Autodesk Inventor part; units mm, degrees
ref_plane "YZ Plane" through (0, 0, 0) normal (1, 0, 0) x (0, 1, 0)
ref_plane "XZ Plane" through (0, 0, 0) normal (0, 1, 0) x (-1, 0, 0)
ref_plane "XY Plane" through (0, 0, 0) normal (0, 0, 1) x (1, 0, 0)
sketch "Szkic1" plane through (0, 0, 0) normal (0, 0, 1) x (1, 0, 0)
  line L0 (9.9, 0) -> (9.9, 2)
  line L1 (9.9, 2) -> (1.4, 2)
  line L2 (1.4, 2) -> (0.4, 3)
  line L3 (0.4, 3) -> (0, 3)
  arc A0 (0, 3) -> (-1.4487, 0) centre (8.1549, -2.7877) ccw
  line L4 (-1.1, 1) -> (9.9, 1) construction
  line L5 (-1.4487, 0) -> (0, 0)
  line L6 (9.9, 0) -> (0, 0)
  dimension "d1" = 11
  dimension "d2" = 1.1
  dimension "d3" = 10
  dimension "d9" = 2.5
  dimension "d10" = 45
  dimension "d11" = 1
  dimension "d12" = 3
revolve "Obrót1" add sketch "Szkic1" angle 360 about axis through (9.9, 0, 0) along (-1, 0, 0)
sketch "Szkic2" plane through (9.9, 0, 0) normal (1, 0, 0) x (0, 0, -1)
  circle A0 centre (0, 0) radius 2
  line L0 (-1.1303, -1.65) -> (1.1303, -1.65)
  line L1 (1.65, -1.1303) -> (1.65, 1.1303)
  line L2 (1.1303, 1.65) -> (-1.1303, 1.65)
  line L3 (-1.65, 1.1303) -> (-1.65, -1.1303)
  line L4 (-1.65, -1.65) -> (1.65, 1.65) construction
  line L5 (1.65, -1.65) -> (-1.65, 1.65) construction
  dimension "d14" = 3.3
  dimension "d15" = 3.3
extrude "Wyciągnięcie proste2" cut sketch "Szkic2" against normal blind 4 contours A0 L1 | L2 A0 | A0 L0 | L3 A0
sketch "Szkic3" plane through (9.9, -1.1303, -1.65) normal (1, 0, 0) x (0, 0, -1)
  line L0 (-2.7803, -0.5197) -> (-0.5197, -0.5197)
  arc A0 (-0.5197, -0.5197) -> (0, 0) centre (-1.65, 1.1303) ccw
  line L1 (0, 0) -> (0, 2.2605)
  arc A1 (0, 2.2605) -> (-0.5197, 2.7803) centre (-1.65, 1.1303) ccw
  line L2 (-0.5197, 2.7803) -> (-2.7803, 2.7803)
  arc A2 (-2.7803, 2.7803) -> (-3.3, 2.2605) centre (-1.65, 1.1303) ccw
  line L3 (-3.3, 2.2605) -> (-3.3, 0)
  arc A3 (-3.3, 0) -> (-2.7803, -0.5197) centre (-1.65, 1.1303) ccw
hole "Otwór1" at (9.9, 0, 0) direction (-1, 0, 0) diameter 1.8 end through all counterbore diameter 2.4 counterbore depth 2.5
chamfer "Faza1" distance 0.25 angle 45 1 edges at (7.4, 0, 0.9)
chamfer "Faza2" distance 0.25 angle 45 2 edges at (-1.1403, -0.6363, 0.6365) (-1.1403, 0.6364, -0.6364)
sketch "Szkic5" plane through (0, 0, 0) normal (0, 1, 0) x (-1, 0, 0)
  line L0 (0, 3) -> (0, -3) construction
  line L1 (1.0546, -0.55) -> (-0.0454, -0.55)
  line L2 (-0.0454, -0.55) -> (-0.0454, 0.55)
  line L3 (-0.0454, 0.55) -> (1.0546, 0.55)
  line L4 (1.0546, 0.55) -> (1.0546, -0.55)
  line L5 (1.0546, -0.55) -> (-0.0454, 0.55) construction
  line L6 (-0.0454, -0.55) -> (1.0546, 0.55) construction
  point P0 (0, 0)
  point P1 (0.5046, 0)
  dimension "d33" = 1.1
  dimension "d34" = 1.1
extrude "Wyciągnięcie proste3" cut sketch "Szkic5" along normal through all both and the other way through all
thread "Gwint1"
properties part number "Nypel_szprychy" material "Aluminium AW-7020"
Here's how the part is built. I have some questions about the finished solid (model axes, mm). A direction names the side the tool comes from. Round coordinates to 2 decimals unless told otherwise and drop trailing zeros. Order: outer loops, then holes, each group sorted by start corner. A loop starts at its lowest first (then second) coordinate and runs counter-clockwise, first axis right, second up. Notation, with made-up numbers: M -30.5,60.25 L 8.5,60.25 A22 cw 8.5,95.25 Z; hole C 46.5,-24.75 d10. An arc over 180 degrees is marked long. Answer in a Markdown table with one row per item.
Item 1: Imagine slicing it at B-B, the plane x = 3.25. Write out the boundary of the cut face in (y, z), and give its area (3 significant figures).
A:
| item | result |
|---|---|
| outline | C 0,0 d4; hole C 0,0 d1.8 |
| area | 10.0 mm2 |
Item 2: Imagine slicing it at C-C, the plane x = 9. Write out the boundary of the cut face in (y, z).
A:
| item | result |
|---|---|
| outline | M -1.65,-1.13 A2 ccw -1.13,-1.65 L 1.13,-1.65 A2 ccw 1.65,-1.13 L 1.65,1.13 A2 ccw 1.13,1.65 L -1.13,1.65 A2 ccw -1.65,1.13 Z; hole C 0,0 d2.4 |
Item 3: If I drill on L1, parallel to Z at x = 7, y = 0; L2, parallel to Z at x = 8.25, y = 0; L3, parallel to Y at x = 5, z = 0, over which ranges is the centre line in solid material (lowest first)? Write a range as from..to.
A:
| item | result |
|---|---|
| L1 | z = -1.65..-0.9, 0.9..1.65 |
| L2 | z = -1.65..-1.2, 1.2..1.65 |
| L3 | y = -2..-0.9, 0.9..2 |
Item 4: Imagine slicing it at A-A, the plane z = 0. Write out the boundary of the cut face in (x, y), and give its area (3 significant figures).
A:
| item | result |
|---|---|
| outline | M 0.05,-3 L 0.4,-3 L 1.4,-2 L 5.9,-2 L 5.9,-1.65 L 9.9,-1.65 L 9.9,-1.2 L 7.4,-1.2 L 7.4,-1.15 L 7.15,-0.9 L 0.05,-0.9 Z; M 0.05,0.9 L 7.15,0.9 L 7.4,1.15 L 7.4,1.2 L 9.9,1.2 L 9.9,1.65 L 5.9,1.65 L 5.9,2 L 1.4,2 L 0.4,3 L 0.05,3 Z |
| area | 19.0 mm2 |
Item 5: I'm going to push flat-ended pins straight in: pin 1 (0.7 mm diameter, centred on y = -0.5, z = 0.5, fed in from +X); pin 2 (2.5 mm diameter, centred on x = 9, z = -0.5, fed in from -Y); pin 3 (0.9 mm diameter, centred on x = -0.5, y = -1.5, fed in from +Z). Where does each tip first touch, or does it pass through?
A:
| item | result |
|---|---|
| pin 1 | stops at x = 7.31 |
| pin 2 | stops at y = -1.65 |
| pin 3 | stops at z = 2.56 |
Item 6: For faces 5 (the face through (8, 0, 1.65)), 6 (the face through (-0.4, 1.6, 0.55)), 7 (the face through (8, 0, -1.65)), which set-ups out of +Z, -Z, +X, -X, +Y, -Y let a thin tool reach every point of the face, with its end or its side?
A:
| item | result |
|---|---|
| face 5 | +Z, +X, +Y, -Y |
| face 6 | -X, +Y, -Y |
| face 7 | -Z, +X, +Y, -Y |
Item 7: Thinking about a two-plate mould opening in Y: for faces 1 (the face through (8, -1.65, 0)), 2 (the face through (-0.4, -1.6, -0.55)), 3 (the face through (5, -2, 0)), 4 (the face through (8.63, -1.01, -0.65)), which applies, +Y half, -Y half, draft (parallel to the pull), parting line (faces both ways), or undercut?
A:
| item | result |
|---|---|
| face 1 | -Y half |
| face 2 | draft |
| face 3 | parting line |
| face 4 | undercut |
Item 8: Imagine slicing it at D-D, the plane x = 7. Write out the boundary of the cut face in (y, z), and give its area (3 significant figures).
A:
| item | result |
|---|---|
| outline | M -1.65,-1.13 A2 ccw -1.13,-1.65 L 1.13,-1.65 A2 ccw 1.65,-1.13 L 1.65,1.13 A2 ccw 1.13,1.65 L -1.13,1.65 A2 ccw -1.65,1.13 Z; hole C 0,0 d1.8 |
| area | 7.87 mm2 |
